from build123d import *

# Parameters (mm, degrees)
SKETCH1_W                      = 50
SKETCH1_H                      = 15
BOSS_EXTRUDE1_DEPTH            = 3
SKETCH2_W                      = 35
SKETCH2_H                      = 3
BOSS_EXTRUDE2_DEPTH            = 47
SKETCH3_W                      = 30.36922738
SKETCH3_H                      = 3
BOSS_EXTRUDE3_DEPTH            = 15
SKETCH4_W                      = 30.36922738
SKETCH4_H                      = 3
BOSS_EXTRUDE4_DEPTH            = 15
CUT_EXTRUDE1_DEPTH             = 42.776189391
F_4_0_4_DIAMETER_HOLE1_D       = 3.5
F_4_0_4_DIAMETER_HOLE1_DEPTH   = 3
F_3_2_3_2_DIAMETER_HOLE1_D     = 3.2
F_3_2_3_2_DIAMETER_HOLE1_DEPTH = 11
CUT_EXTRUDE2_START             = -15
SKETCH14_W                     = 8
SKETCH14_H                     = 3
CUT_EXTRUDE2_DEPTH             = 72.471231614
SKETCH15_W                     = 17.327316674
SKETCH15_H                     = 3.5
CUT_EXTRUDE3_DEPTH             = 10
BOSS_EXTRUDE5_DEPTH            = 5


with BuildPart() as part:
    # Sketch1 → Boss-Extrude1 (new body)
    with BuildSketch(Plane.XY.offset(25)):
        with Locations((0, -0.5)):
            Rectangle(SKETCH1_W, SKETCH1_H)
    extrude(amount=-BOSS_EXTRUDE1_DEPTH)

    # Sketch2 → Boss-Extrude2 (add)
    with BuildSketch(Plane(origin=(0, 0, 22), x_dir=(-1, 0, 0), z_dir=(0, 0, -1))):
        with Locations((0, 1.5)):
            Rectangle(SKETCH2_W, SKETCH2_H)
    extrude(amount=BOSS_EXTRUDE2_DEPTH)

    # Sketch3 → Boss-Extrude3 (add)
    with BuildSketch(Plane(origin=(17.5, 0, 0), x_dir=(0, 0, -1), z_dir=(1, 0, 0))):
        with Locations((9.81538631, 1.5)):
            Rectangle(SKETCH3_W, SKETCH3_H)
    extrude(amount=BOSS_EXTRUDE3_DEPTH)

    # Sketch4 → Boss-Extrude4 (add)
    with BuildSketch(Plane.ZY.offset(17.5)):
        with Locations((-9.81538631, 1.5)):
            Rectangle(SKETCH4_W, SKETCH4_H)
    extrude(amount=BOSS_EXTRUDE4_DEPTH)

    # Sketch5 → Cut-Extrude1 (cut, through all)
    with BuildSketch(Plane.XZ):
        Polygon((17.5, -25), (17.5, -17), (13.6, -17), (13.6, -3.25), (5.6, -3.25), (5.6, -17), (-5.6, -17), (-5.6, -3.25), (-13.6, -3.25), (-13.6, -17), (-17.5, -17), (-17.5, -25), align=None)
    extrude(amount=-CUT_EXTRUDE1_DEPTH, mode=Mode.SUBTRACT)

    # Ø4.0 (4) Diameter Hole1
    with Locations(Plane.XY.offset(25)):
        with Locations((22, -0.5), (-22, -0.5)):
            Hole(F_4_0_4_DIAMETER_HOLE1_D / 2, depth=F_4_0_4_DIAMETER_HOLE1_DEPTH)

    # Ø3.2 (3.2) Diameter Hole1
    with Locations(Plane(origin=(0, 3, 0), x_dir=(1, 0, 0), z_dir=(0, 1, 0))):
        with Locations((-27.5, -1), (27.5, -1)):
            Hole(F_3_2_3_2_DIAMETER_HOLE1_D / 2, depth=F_3_2_3_2_DIAMETER_HOLE1_DEPTH)

    # Sketch14 → Cut-Extrude2 (cut, through all)
    with BuildSketch(Plane(origin=(-17.5, 0, 0), x_dir=(0, 0, -1), z_dir=(1, 0, 0)).offset(CUT_EXTRUDE2_START)):
        with Locations((21, 1.5)):
            Rectangle(SKETCH14_W, SKETCH14_H)
    extrude(amount=CUT_EXTRUDE2_DEPTH, mode=Mode.SUBTRACT)

    # Sketch15 → Cut-Extrude3 (cut)
    with BuildSketch(Plane(origin=(0, 3, 0), x_dir=(1, 0, 0), z_dir=(0, 1, 0))):
        Rectangle(SKETCH15_W, SKETCH15_H)
    extrude(amount=-CUT_EXTRUDE3_DEPTH, mode=Mode.SUBTRACT)

    # Sketch17 → Boss-Extrude5 (add)
    with BuildSketch(Plane(origin=(17.5, 0, 0), x_dir=(0, 0, -1), z_dir=(1, 0, 0))):
        Polygon((-22, -3.655953394), (-11.540106588, 0), (-22, 0), align=None)
    boss_extrude5 = extrude(amount=-BOSS_EXTRUDE5_DEPTH)

    # Mirror1: Boss-Extrude5 across plane
    add(boss_extrude5.mirror(Plane(origin=(0, 0, 0), x_dir=(0, 0, 1), z_dir=(1, 0, 0))))


solid = part.part
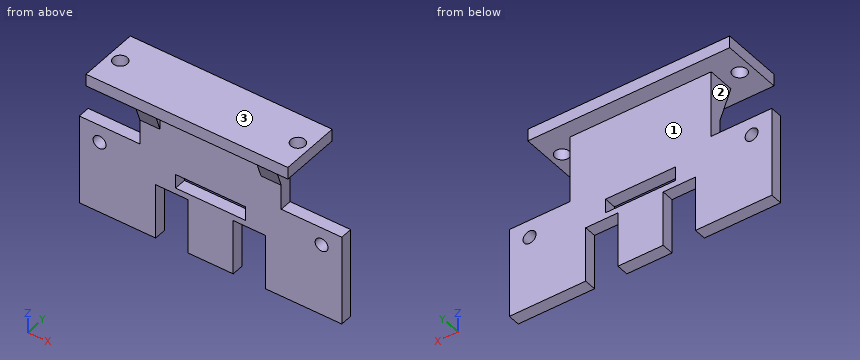
Can you work these out from the model? Positions are in its coordinate system, mm. Face numbers are marked on the shaded views. Round coordinates to 2 decimals unless told otherwise and drop trailing zeros. Loops run counter-clockwise (first coordinate to the right, second up) from the corner with the lowest first, then second, coordinate; pieces in that order, holes last. Notation, with made-up numbers: (-32, 63) - (-21, 63) arc R6 cw to (-21, 73) - close; hole circle Ø7 at (69, 71.5). An arc over 180 degrees is marked (long way). Answer in a Markdown table with one row per item. Add a question column.
Q1. For pin 1 Ø2 at (y, z) = (3, 16.5) entering from +X; pin 2 Ø6 at (x, z) = (5, 8) entering from -Y; pin 3 Ø11.5 at (x, z) = (9.5, 10.5) entering from +Y; pin 4 Ø7.5 at (x, y) = (12.5, 0.5) entering from -Z, each with a flat end and sliding along its axis, tell me the tip position at first contact or that it passes through.
Q2. I need wall thicknesses on L1, parallel to Z at x = -27.5, y = 1; L2, parallel to Y at x = -22, z = 23.6; L3, parallel to Y at x = 2, z = 3.5. Which ranges of each line are inside material? Lowest first, please.
Q3. I want a section at D-D on x = -23. List the corners of the cut face in (y, z) for me, and give its area (3 significant figures).
Q4. I want a section at B-B on z = 1. List the corners of the cut face in (x, y) for me.
Q5. I want a section at A-A on x = 27.5. List the corners of the cut face in (y, z) for me, and give its area (3 significant figures).
Q6. We'd pull the mould along Z, two halves only. Please class the marked faces 1, 2 and 3: pulls with the +Z half, pulls with the -Z half, needs draft (parallel to the pull), parting line crosses it, or undercut.
Q7. I want a section at C-C on y = 2.25. List the corners of the cut face in (x, z) for me.
A:
| question | item | result |
|---|---|---|
| 1 | pin 1 | x = 17.5 |
| 1 | pin 2 | y = 0 |
| 1 | pin 3 | y = 3 |
| 1 | pin 4 | z = -17 |
| 2 | L1 | -17 to -0.6, 2.6 to 5.37 |
| 2 | L2 | -8 to -2.25, 1.25 to 7 |
| 2 | L3 | 0 to 3 |
| 3 | outline | (-8, 22) - (-1.94, 22) - (-1.94, 25) - (-8, 25) - close; (0, -17) - (3, -17) - (3, 5.37) - (0, 5.37) - close; (0.94, 22) - (7, 22) - (7, 25) - (0.94, 25) - close |
| 3 | area | 103 mm^2 |
| 4 | outline | (-32.5, 0) - (-29.1, 0) - (-29.1, 3) - (-32.5, 3) - close; (-25.9, 0) - (-8.66, 0) - (-8.66, 3) - (-25.9, 3) - close; (8.66, 0) - (25.9, 0) - (25.9, 3) - (8.66, 3) - close; (29.1, 0) - (32.5, 0) - (32.5, 3) - (29.1, 3) - close |
| 5 | outline | (0, -17) - (3, -17) - (3, -0.6) - (0, -0.6) - close; (0, 2.6) - (3, 2.6) - (3, 5.37) - (0, 5.37) - close |
| 5 | area | 57.5 mm^2 |
| 6 | face 1 | needs draft |
| 6 | face 2 | undercut |
| 6 | face 3 | pulls with the +Z half |
| 7 | outline | (-32.5, -17) - (-13.6, -17) - (-13.6, -3.25) - (-5.6, -3.25) - (-5.6, -17) - (5.6, -17) - (5.6, -3.25) - (13.6, -3.25) - (13.6, -17) - (32.5, -17) - (32.5, 5.37) - (17.5, 5.37) - (17.5, 22) - (25, 22) - (25, 25) - (-25, 25) - (-25, 22) - (-17.5, 22) - (-17.5, 5.37) - (-32.5, 5.37) - close; hole circle Ø3.2 at (-27.5, 1); hole (-8.66, -1.75) - (8.66, -1.75) - (8.66, 1.75) - (-8.66, 1.75) - close; hole circle Ø3.2 at (27.5, 1) |
